Geometry: final body of the model. Coordinates: model frame, mm. Give positions to 0.01 mm unless a question says otherwise; leave off trailing zeros. Write each loop counter-clockwise with the first axis right and the second up, starting at its lowest first coordinate (ties: lowest second). Pieces come first, ordered by that corner, then holes. Notation, with made-up numbers: (83, 61) -> (136, 61) arc R23 cw to (136, 87) -> close; hole circle Ø3 at (-1.5, 55). An arc over 180 degrees is marked (long way). Use CSV: the item, a comma, the result in double quotes. Start each with the question number.
1) Material intervals for line 1 (X direction, y = -7.25, z = 1.4); line 2 (X direction, y = -22.25, z = 1); line 3 (Y direction, x = -9, z = 0.75), sorted ascending. Write a range as [from, to].
2) Contact query for a flat-ended pin moving along its axis: P1, Ø2.5, axis at x = -9, y = -7.5, coming from the -Z side. Output: stop coordinate, or through.
3) Section D-D (z = 2.55). Count the separate pieces of the cut face and the enclosed holes in it, plus the area to 3 significant figures.
4) Section B-B (x = -9). Output: boundary loops of the cut face in (y, z), plus the area to 3 significant figures.
5) Section A-A (y = -15). Output: boundary loops of the cut face in (x, z), plus the area to 3 significant figures.
6) Section C-C (y = -7.5). Output: boundary loops of the cut face in (x, z).
```python
from build123d import *

# Parameters (mm, degrees)
EXTRUDE_1_DEPTH     = 3
SKETCH_2_W          = 8
SKETCH_2_H          = 4.5
SKETCH_2_H_2        = 13.5
CUT_EXTRUDE_1_DEPTH = 3
SKETCH_4_W          = 76.2
SKETCH_4_H          = 6
CUT_EXTRUDE_2_DEPTH = 3
SKETCH_6_W          = 12
SKETCH_6_H          = 6
EXTRUDE_2_DEPTH     = 3
FILLET_1_R          = 1.5
SKETCH_7_R          = 1.5
CUT_EXTRUDE_3_DEPTH = 10


with BuildPart() as part:
    # 草图1 → 凸台-拉伸1 (new body)
    with BuildSketch(Plane.XY):
        Polygon((18, 0), (18, -24), (78.2, -24), (78.2, 0), (96.2, 0), (96.2, -30), (0, -30), (0, 0), align=None)
        with BuildLine():
            Line((3, -4.5), (7, -4.5))
            ThreePointArc((7, -4.5), (8, -5.5), (7, -6.5))
            Line((7, -6.5), (7, -8.5))
            ThreePointArc((7, -8.5), (8, -9.5), (7, -10.5))
            Line((7, -10.5), (3, -10.5))
            ThreePointArc((3, -10.5), (2, -9.5), (3, -8.5))
            Line((3, -8.5), (3, -6.5))
            ThreePointArc((3, -6.5), (2, -5.5), (3, -4.5))
        make_face(mode=Mode.SUBTRACT)
        with BuildLine():
            Line((89.2, -6.5), (89.2, -8.5))
            ThreePointArc((89.2, -8.5), (88.2, -9.5), (89.2, -10.5))
            Line((89.2, -10.5), (93.2, -10.5))
            ThreePointArc((93.2, -10.5), (94.2, -9.5), (93.2, -8.5))
            Line((93.2, -8.5), (93.2, -6.5))
            ThreePointArc((93.2, -6.5), (94.2, -5.5), (93.2, -4.5))
            Line((93.2, -4.5), (89.2, -4.5))
            ThreePointArc((89.2, -4.5), (88.2, -5.5), (89.2, -6.5))
        make_face(mode=Mode.SUBTRACT)
    extrude(amount=EXTRUDE_1_DEPTH)

    # 草图2 → 切除-拉伸1 (cut)
    with BuildSketch(Plane.XY.offset(3)):
        with Locations((14, -2.25)):
            Rectangle(SKETCH_2_W, SKETCH_2_H)
        with Locations((14, -17.25)):
            Rectangle(SKETCH_2_W, SKETCH_2_H_2)
        with Locations((82.2, -17.25)):
            Rectangle(SKETCH_2_W, SKETCH_2_H_2)
        with Locations((82.2, -2.25)):
            Rectangle(SKETCH_2_W, SKETCH_2_H)
    extrude(amount=-CUT_EXTRUDE_1_DEPTH, mode=Mode.SUBTRACT)

    # 草图4 → 切除-拉伸2 (cut)
    with BuildSketch(Plane.XY.offset(3)):
        with Locations((48.1, -7.5)):
            Rectangle(SKETCH_4_W, SKETCH_4_H)
    extrude(amount=-CUT_EXTRUDE_2_DEPTH, mode=Mode.SUBTRACT)

    # 草图6 → 凸台-拉伸2 (add)
    with BuildSketch(Plane.XY.offset(3)):
        with Locations((102.2, -7.5)):
            Rectangle(SKETCH_6_W, SKETCH_6_H)
        with Locations((-6, -7.5)):
            Rectangle(SKETCH_6_W, SKETCH_6_H)
    extrude(amount=-EXTRUDE_2_DEPTH)

    # 圆角1
    fillet_1_edges = [part.edges().sort_by_distance(p)[0] for p in [
        (10, -24, 1.5),
        (10, 0, 1.5),
        (0, 0, 1.5),
        (96.2, 0, 1.5),
        (96.2, -30, 1.5),
        (0, -30, 1.5),
        (96.2, -10.5, 1.5),
        (96.2, -4.5, 1.5),
        (108.2, -4.5, 1.5),
        (108.2, -10.5, 1.5),
        (-12, -4.5, 1.5),
        (0, -4.5, 1.5),
        (0, -10.5, 1.5),
        (-12, -10.5, 1.5),
        (86.2, 0, 1.5),
        (86.2, -24, 1.5),
    ]]
    fillet(fillet_1_edges, radius=FILLET_1_R)

    # 草图7 → 切除-拉伸3 (cut)
    with BuildSketch(Plane.XY.offset(3)):
        with Locations((-9, -7.5)):
            Circle(SKETCH_7_R)
        with Locations((105.2, -7.5)):
            Circle(SKETCH_7_R)
    extrude(amount=-CUT_EXTRUDE_3_DEPTH, mode=Mode.SUBTRACT)


solid = part.part
```
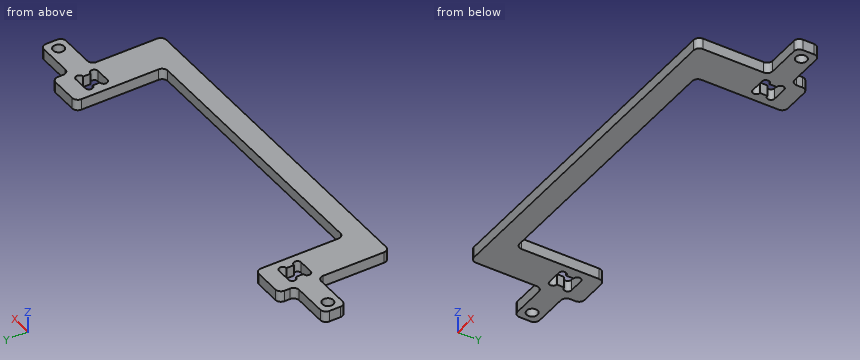
Answers follow:
1,line 1,"x = [-12, -10.48], [-7.52, 3], [7, 10], [86.2, 89.2], [93.2, 103.72], [106.68, 108.2]"
1,line 2,"x = [0, 10], [86.2, 96.2]"
1,line 3,"y = [-10.5, -9], [-6, -4.5]"
2,P1,"passes through"
3,separate pieces,"1"
3,enclosed holes,"4"
3,area,"1,120 mm^2"
4,outline,"(-10.5, 0) -> (-9, 0) -> (-9, 3) -> (-10.5, 3) -> close; (-6, 0) -> (-4.5, 0) -> (-4.5, 3) -> (-6, 3) -> close"
4,area,"9.00 mm^2"
5,outline,"(0, 0) -> (10, 0) -> (10, 3) -> (0, 3) -> close; (86.2, 0) -> (96.2, 0) -> (96.2, 3) -> (86.2, 3) -> close"
5,area,"60.0 mm^2"
6,outline,"(-12, 0) -> (-10.5, 0) -> (-10.5, 3) -> (-12, 3) -> close; (-7.5, 0) -> (3, 0) -> (3, 3) -> (-7.5, 3) -> close; (7, 0) -> (10, 0) -> (10, 3) -> (7, 3) -> close; (86.2, 0) -> (89.2, 0) -> (89.2, 3) -> (86.2, 3) -> close; (93.2, 0) -> (103.7, 0) -> (103.7, 3) -> (93.2, 3) -> close; (106.7, 0) -> (108.2, 0) -> (108.2, 3) -> (106.7, 3) -> close"
